from build123d import *

# Parameters (mm, degrees)
SKETCH1_R                  = 152.4
BOSS_EXTRUDE1_DEPTH        = 19.05
SKETCH5_R                  = 55
CUT_EXTRUDE1_DEPTH         = 217.366407975
F_3_8_CLEARANCE_HOLE1_D    = 9.8044
NIPPLE_SOCKET_CLEARANCE_BY = 0.5


with BuildPart() as part:
    # Sketch1 → Boss-Extrude1 (new body)
    with BuildSketch(Plane.XY):
        with Locations(Location((0, 0, 0), (0, 0, 180))):
            Circle(SKETCH1_R)
    extrude(amount=BOSS_EXTRUDE1_DEPTH)

    # Sketch5 → Cut-Extrude1 (cut, through all)
    with BuildSketch(Plane(origin=(0, 0, 0), x_dir=(-1, 0, 0), z_dir=(0, 0, -1))):
        Circle(SKETCH5_R)
    extrude(amount=-CUT_EXTRUDE1_DEPTH, mode=Mode.SUBTRACT)

    # 3/8 Clearance Hole1 (through all)
    with Locations(Plane.XY.offset(19.05)):
        with Locations((25.523973959, -61.673028045), (61.624734649, -25.605296339), (61.648089668, 25.425534023), (25.580357962, 61.526294713), (-25.450472399, 61.549649732), (-61.55123309, 25.481918026), (-61.574588109, -25.548912335), (-25.506856403, -61.649673026)):
            Hole(F_3_8_CLEARANCE_HOLE1_D / 2)

    # nipple-socket-clearance: a curved face moved inward by 0.5
    add(Solid.thicken(part.faces().sort_by_distance((55, 0, 9.525))[0], -NIPPLE_SOCKET_CLEARANCE_BY), mode=Mode.SUBTRACT)


solid = part.part
Work out the finished part from the listing and answer in its coordinate system (mm). Coordinates: 2 decimals unless noted, no trailing zeros. Write each loop counter-clockwise with the first axis right and the second up, starting at its lowest first coordinate (ties: lowest second). Pieces come first, ordered by that corner, then holes. Notation, with made-up numbers: M 53,0 L 86,0 A27 cw 86,36 Z; hole C 18,87.5 d6. An arc over 180 degrees is marked long. Write item = value, one per line.
1. Flat-ended cylindrical pins translate along their axes: pin 1 (6 mm diameter, centred on x = -61.55, y = 25.48, fed in from -Z); pin 2 (6 mm diameter, centred on x = 5, z = 13, fed in from +Y); pin 3 (6 mm diameter, centred on x = -113.5, z = 14.5, fed in from +Y); pin 4 (6 mm diameter, centred on x = -120.5, z = 4.5, fed in from -Y). Find the tip coordinate at first contact, or state that the pin passes through.
Solution:
pin_1 = through
pin_2 = 152.39
pin_3 = 104.95
pin_4 = -97.05
2. The part is cut by section D-D (y = -97). Determine the outline of the cut face in (x, z).
Solution:
outline = M -117.54,0 L 117.54,0 L 117.54,19.05 L -117.54,19.05 Z
3. The part is cut by section A-A (y = 0). Determine the outline of the cut face in (x, z), then the cut area to 3 significant figures.
Solution:
outline = M -152.4,0 L -55.5,0 L -55.5,19.05 L -152.4,19.05 Z; M 55.5,0 L 152.4,0 L 152.4,19.05 L 55.5,19.05 Z
area = 3,690 mm2
4. Determine the mould class of faces 1 (the face through (56.972, 26.898, 9.392)), 2 (the face through (-66, -2, 19.05)), 3 (the face through (33.037, 148.776, 9.392)) for opening direction Y: released by +Y, released by -Y, zero draft, split by the parting line, or undercut.
Solution:
face_1 = undercut
face_2 = zero draft
face_3 = split by the parting line
5. Straight lines are drawn through the part: line 1 (Y direction, x = -28.5, z = 15.75); line 2 (Y direction, x = 0, z = 14); line 3 (X direction, y = 16, z = 11). For each, find the intervals that lie inside material, in ascending order. Write a range as from..to.
Solution:
line_1 = -149.71..-65.53, -57.77..-47.62, 47.62..57.71, 65.39..149.71
line_2 = -152.4..-55.5, 55.5..152.4
line_3 = -151.56..-53.14, 53.14..151.56
6. The part is cut by section C-C (z = 15.5). State how many separate pieces and enclosed holes the cut face has, then the cut area to 3 significant figures.
Solution:
separate_pieces = 1
enclosed_holes = 9
area = 62,700 mm2
